Source: CAD feature listing. Evaluate the final solid. Frame: model axes, mm. A direction names the side the tool comes from. Give positions to 0.01 mm unless a question says otherwise; leave off trailing zeros. Order: outer loops, then holes, each group sorted by start corner. A loop starts at its lowest first (then second) coordinate and runs counter-clockwise, first axis right, second up. Notation, with made-up numbers: M 89.25,23 L 117.25,23 A30 cw 117.25,51 Z; hole C -40,-19.5 d6. An arc over 180 degrees is marked long. Answer as a JSON object with one key per item and string values. Group by question number.
1. Section query C-C (z = 0). Output: boundary loops of the cut face in (x, y), plus the area to 3 significant figures.
2. Section query B-B (y = 36). Output: boundary loops of the cut face in (x, z), plus the area to 3 significant figures.
3. Material intervals for L1, parallel to X at y = 20.5, z = -39; L2, parallel to Z at x = 0, y = 6, sorted ascending. Write a range as [from, to].
4. Set-up query: faces 5 (the flat face through (-65, 10.15, -44)), 6 (the flat face through (101.6, 39, 1)). Return all of +Z, -Z, +X, -X, +Y, -Y with unobstructed straight access to the full face (end or side cutting, diameter ignored); none if empty.
5. Section query A-A (x = 0). Output: boundary loops of the cut face in (y, z), plus the area to 3 significant figures.
6. Pull-direction query (Z, two-part tool) for faces 1 (the flat face through (-1, 46, -95.25)), 2 (the flat face through (-8, 80, 97)), 3 (the flat face through (-1, 39, 101.6)), 4 (the flat face through (95.25, 46, 1)); classes: +Z half, -Z half, draft (parallel to the pull), parting line (faces both ways), or undercut.
7. Section query D-D (y = 6). Output: boundary loops of the cut face in (x, z).
from build123d import *

# Parameters (mm, degrees)
SKETCH1_W           = 203.2
SKETCH1_H           = 203.2
BOSS_EXTRUDE1_DEPTH = 80
SKETCH3_R           = 75.5
CUT_EXTRUDE1_DEPTH  = 80
SKETCH4_W           = 190.5
SKETCH4_H           = 190.5
CUT_EXTRUDE2_DEPTH  = 69.85


with BuildPart() as part:
    # Sketch1 → Boss-Extrude1 (new body)
    with BuildSketch(Plane(origin=(0, 0, 0), x_dir=(1, 0, 0), z_dir=(0, 1, 0))):
        Rectangle(SKETCH1_W, SKETCH1_H)
    extrude(amount=BOSS_EXTRUDE1_DEPTH)

    # Sketch3 → Cut-Extrude1 (cut)
    with BuildSketch(Plane(origin=(0, 80, 0), x_dir=(1, 0, 0), z_dir=(0, 1, 0))):
        Circle(SKETCH3_R)
    extrude(amount=-CUT_EXTRUDE1_DEPTH, mode=Mode.SUBTRACT)

    # Sketch4 → Cut-Extrude2 (cut)
    with BuildSketch(Plane(origin=(0, 80, 0), x_dir=(1, 0, 0), z_dir=(0, 1, 0))):
        Rectangle(SKETCH4_W, SKETCH4_H)
    extrude(amount=-CUT_EXTRUDE2_DEPTH, mode=Mode.SUBTRACT)


solid = part.part
Answer sheet:
{
 "1": {"outline": "M -101.6,0 L -75.5,0 L -75.5,10.15 L -95.25,10.15 L -95.25,80 L -101.6,80 Z; M 75.5,0 L 101.6,0 L 101.6,80 L 95.25,80 L 95.25,10.15 L 75.5,10.15 Z", "area": "1,420 mm^2"},
 "2": {"outline": "M -101.6,-101.6 L 101.6,-101.6 L 101.6,101.6 L -101.6,101.6 Z; hole M -95.25,-95.25 L 95.25,-95.25 L 95.25,95.25 L -95.25,95.25 Z", "area": "5,000 mm^2"},
 "3": {"L1": "[-101.6, -95.25], [95.25, 101.6]", "L2": "[-101.6, -75.5], [75.5, 101.6]"},
 "4": {"face 5": "+Y", "face 6": "+Z, -Z, +X, +Y, -Y"},
 "5": {"outline": "M 0,-101.6 L 80,-101.6 L 80,-95.25 L 10.15,-95.25 L 10.15,-75.5 L 0,-75.5 Z; M 0,75.5 L 10.15,75.5 L 10.15,95.25 L 80,95.25 L 80,101.6 L 0,101.6 Z", "area": "1,420 mm^2"},
 "6": {"face 1": "undercut", "face 2": "draft", "face 3": "+Z half", "face 4": "undercut"},
 "7": {"outline": "M -101.6,-101.6 L 101.6,-101.6 L 101.6,101.6 L -101.6,101.6 Z; hole C 0,0 d151"}
}
